Can you work these out from the model? Positions are in its coordinate system, mm. A direction names the side the tool comes from. Give positions to 0.01 mm unless a question says otherwise; leave off trailing zeros. Write each loop counter-clockwise with the first axis right and the second up, starting at its lowest first coordinate (ties: lowest second). Pieces come first, ordered by that corner, then holes.
```python
from build123d import *

# Parameters (mm, degrees)
F1_DEPTH = 3.5
F3_DEPTH = 2
F4_R     = 1.9
F5_DEPTH = 25
F7_DEPTH = 25
F9_DEPTH = 25


with BuildPart() as f1:
    # F0 (on Top) → F1 (new body)
    with BuildSketch(Plane.XY):
        with BuildLine():
            Line((-5, 0), (-5, -3))
            Line((-5, -3), (2, -3))
            ThreePointArc((2, -3), (4.12132, -2.12132), (5, 0))
            Line((5, 0), (5, 3))
            Line((5, 3), (-2, 3))
            ThreePointArc((-2, 3), (-4.12132, 2.12132), (-5, 0))
        make_face()
    extrude(amount=F1_DEPTH)

    # F2 (on face) → F3 (join)
    with BuildSketch(Plane.XY.offset(3.5)):
        with BuildLine():
            Line((3, 0), (3, 3))
            Line((3, 3), (0, 3))
            ThreePointArc((0, 3), (-2.12132, 2.12132), (-3, 0))
            Line((-3, 0), (-3, -3))
            Line((-3, -3), (0, -3))
            ThreePointArc((0, -3), (2.12132, -2.12132), (3, 0))
        make_face()
    extrude(amount=F3_DEPTH)

    # F4 (on face) → F5 (cut)
    with BuildSketch(Plane.XY.offset(5.5)):
        Circle(F4_R)
    extrude(amount=-F5_DEPTH, mode=Mode.SUBTRACT)

    # F6 (on face) → F7 (cut)
    with BuildSketch(Plane.XZ.offset(3)):
        Polygon((-2.5, 0), (-5, 2), (-5, 0), align=None)
    extrude(amount=-F7_DEPTH, mode=Mode.SUBTRACT)

    # F8 (on face) → F9 (cut)
    with BuildSketch(Plane(origin=(0, 3, 0), x_dir=(-1, 0, 0), z_dir=(0, 1, 0))):
        Polygon((-5, 0), (-2.5, 0), (-5, 2), align=None)
    extrude(amount=-F9_DEPTH, mode=Mode.SUBTRACT)


solid = f1.part
```
1) If we mould it in two halves opening along Y, with no side actions, what happens to faces 6 (the face through (2, -1, 5.5)), 7 (the face through (-1.9, 0.08, 2.79)), 8 (the face through (-2.1, 2.14, 4.49)), 9 (the face through (3.69, -2.48, 2.11))? For each: +Y half, -Y half, draft (parallel to the pull), parting line (faces both ways), or undercut.
Values follow:
face 6: draft
face 7: undercut
face 8: +Y half
face 9: -Y half
2) Please list where these lines run through material, in increasing order: L1, parallel to Y at x = 0, z = 3.4; L2, parallel to X at y = -1.25, z = 2.8; L3, parallel to X at y = -1, z = 3.05.
Values follow:
L1: y = -3 to -1.9, 1.9 to 3
L2: x = -5 to -1.43, 1.43 to 4.73
L3: x = -5 to -1.62, 1.62 to 4.83
3) Suppose I cut it at D-D on y = -2.25. Write out the boundary of the cut face in (x, z), plus the area to 3 significant figures.
Values follow:
outline: (-5, 2) - (-2.5, 0) - (2.5, 0) - (3.98, 1.19) - (3.98, 3.5) - (1.98, 3.5) - (1.98, 5.5) - (-3, 5.5) - (-3, 3.5) - (-5, 3.5) - close
area: 38.0 mm2
4) For faces 1 (the face through (-3, -1, 4)), 2 (the face through (1, 2, 0)), 3 (the face through (3, 1, 4)), 4 (the face through (5, 1, 3)), 5 (the face through (2.1, -2.14, 4.49)), which set-ups out of +Z, -Z, +X, -X, +Y, -Y let a thin tool reach every point of the face, with its end or its side?
Values follow:
face 1: +Z, -X, +Y, -Y
face 2: -Z, +X, -X, +Y, -Y
face 3: +Z, +X, +Y, -Y
face 4: +Z, -Z, +X, +Y, -Y
face 5: +Z, +X, -Y
5) Suppose I cut it at A-A on z = 2.35. Write out the boundary of the cut face in (x, y).
Values follow:
outline: (-5, -3) - (2, -3) arc R3 ccw to (5, 0) - (5, 3) - (-2, 3) arc R3 ccw to (-5, 0) - close; hole circle Ø3.8 at (0, 0)
6) Suppose I cut it at C-C on x = -1. Write out the boundary of the cut face in (y, z), plus the area to 3 significant figures.
Values follow:
outline: (-3, 0) - (-1.62, 0) - (-1.62, 5.5) - (-3, 5.5) - close; (1.62, 0) - (3, 0) - (3, 3.5) - (2.83, 3.5) - (2.83, 5.5) - (1.62, 5.5) - close
area: 14.9 mm2
7) Suppose I cut it at B-B on y = -1.25. Write out the boundary of the cut face in (x, z).
Values follow:
outline: (-5, 2) - (-2.5, 0) - (-1.43, 0) - (-1.43, 5.5) - (-3, 5.5) - (-3, 3.5) - (-5, 3.5) - close; (1.43, 0) - (2.5, 0) - (4.73, 1.78) - (4.73, 3.5) - (2.73, 3.5) - (2.73, 5.5) - (1.43, 5.5) - close
8) For pin 1 Ø0.6 at (y, z) = (1, 4.5) entering from +X; pin 2 Ø3.5 at (x, y) = (0, 0) entering from +Z, each with a flat end and sliding along its axis, tell me the tip position at first contact or that it passes through.
Values follow:
pin 1: stops at x = 3
pin 2: passes through
